```python
from build123d import *

# Parameters (mm, degrees)
SKETCH1_W           = 45.78
SKETCH1_H           = 31.61
BOSS_EXTRUDE2_DEPTH = 77.5
SKETCH2_R           = 3.675
CUT_EXTRUDE1_DEPTH  = 25.4
SKETCH3_W           = 39.78
SKETCH3_H           = 47.1
CUT_EXTRUDE3_DEPTH  = 87.772081916


with BuildPart() as part:
    # Sketch1 → Boss-Extrude2 (new body)
    with BuildSketch(Plane(origin=(0, 0, 0), x_dir=(1, 0, 0), z_dir=(0, 1, 0))):
        Rectangle(SKETCH1_W, SKETCH1_H)
    extrude(amount=BOSS_EXTRUDE2_DEPTH)

    # Sketch2 → Cut-Extrude1 (cut)
    with BuildSketch(Plane(origin=(0, 77.5, 0), x_dir=(1, 0, 0), z_dir=(0, 1, 0))):
        with Locations(Location((0, 0, 0), (0, 0, 270))):
            Circle(SKETCH2_R)
    extrude(amount=-CUT_EXTRUDE1_DEPTH, mode=Mode.SUBTRACT)

    # Sketch3 → Cut-Extrude3 (cut, through all)
    with BuildSketch(Plane(origin=(0, 0, -15.805), x_dir=(-1, 0, 0), z_dir=(0, 0, -1))):
        with Locations((0, 23.55)):
            Rectangle(SKETCH3_W, SKETCH3_H)
    extrude(amount=-CUT_EXTRUDE3_DEPTH, mode=Mode.SUBTRACT)


solid = part.part
```
Geometry: final body of the model. Coordinates: model frame, mm. A direction names the side the tool comes from. Give positions to 0.01 mm unless a question says otherwise; leave off trailing zeros. Write each loop counter-clockwise with the first axis right and the second up, starting at its lowest first coordinate (ties: lowest second). Pieces come first, ordered by that corner, then holes.
1. Pin query (flat end, axial travel): P1, Ø9.5, axis at x = -6, z = -5.5, coming from the -Y side; P2, Ø3.5, axis at x = 0.5, z = -0.5, coming from the +Y side; P3, Ø12, axis at x = 17.5, y = 42.5, coming from the +Z side (3 decimals). Return the tip coordinate at first contact, or that it passes through.
2. Section query D-D, the plane y = 66. Return loops of the section in (x, z) (3 decimals).
3. Line query: probe 1 along X at (y, z) = (65, 0) (3 decimals); probe 2 along X at (y, z) = (44.5, -14); probe 3 along Y at (x, z) = (15.5, 8). Output: solid intervals per line, ascending.
4. Draft query along X for faces 4 (the flat face through (-22.89, 38, 0)), 5 (the flat face through (-21, 0, 0)), 6 (the flat face through (19.89, 23, 0)). Return one class per face: released by +X, released by -X, zero draft, split by the parting line, or undercut.
5. Reachability of faces 1 (the flat face through (22.89, 38, 0)), 2 (the flat face through (0, 52.1, 0)), 3 (the flat face through (0, 47.1, 0)) from +Z, -Z, +X, -X, +Y, -Y: full face, straight path, thin tool, end or side. Return the list, or none.
6. Section query B-B, the plane z = 0. Return loops of the section in (x, y) (3 decimals), then the cut area to 3 significant figures.
7. Section query C-C, the plane x = 0. Return loops of the section in (y, z) (3 decimals), then the cut area to 3 significant figures.
8. Section query A-A, the plane y = 8. Return loops of the section in (x, z) (3 decimals).
Computed:
1. P1: stops at y = 47.1
1. P2: stops at y = 52.1
1. P3: stops at z = 15.805
2. outline: (-22.89, -15.805) - (22.89, -15.805) - (22.89, 15.805) - (-22.89, 15.805) - close; hole circle Ø7.35 at (0, 0)
3. probe 1: x = -22.89 to -3.675, 3.675 to 22.89
3. probe 2: x = -22.89 to -19.89, 19.89 to 22.89
3. probe 3: y = 47.1 to 77.5
4. face 4: released by -X
4. face 5: zero draft
4. face 6: undercut
5. face 1: +Z, -Z, +X, +Y, -Y
5. face 2: +Y
5. face 3: +Z, -Z, -Y
6. outline: (-22.89, 0) - (-19.89, 0) - (-19.89, 47.1) - (19.89, 47.1) - (19.89, 0) - (22.89, 0) - (22.89, 77.5) - (3.675, 77.5) - (3.675, 52.1) - (-3.675, 52.1) - (-3.675, 77.5) - (-22.89, 77.5) - close
6. area: 1,490 mm2
7. outline: (47.1, -15.805) - (77.5, -15.805) - (77.5, -3.675) - (52.1, -3.675) - (52.1, 3.675) - (77.5, 3.675) - (77.5, 15.805) - (47.1, 15.805) - close
7. area: 774 mm2
8. outline: (-22.89, -15.805) - (-19.89, -15.805) - (-19.89, 15.805) - (-22.89, 15.805) - close; (19.89, -15.805) - (22.89, -15.805) - (22.89, 15.805) - (19.89, 15.805) - close
